from build123d import *

# Parameters (mm, degrees)
CYLINDER1317_R     = 1
CYLINDER1317_DEPTH = 7
CYLINDER1318_R     = 1
CYLINDER1318_DEPTH = 7
CYLINDER1319_R     = 1
CYLINDER1319_DEPTH = 7
CYLINDER1320_R     = 1
CYLINDER1320_DEPTH = 7
BOX543_W           = 4
BOX543_H           = 11
BOX543_DEPTH       = 4
CYLINDER1293_R     = 2
CYLINDER1293_DEPTH = 11
CYLINDER1292_R     = 3
CYLINDER1292_DEPTH = 6.5
CYLINDER1286_R     = 6
CYLINDER1286_DEPTH = 6.5
CYLINDER1310_R     = 13.75
CYLINDER1310_DEPTH = 5
CYLINDER1291_R     = 5.6
CYLINDER1291_DEPTH = 4.5
CYLINDER1290_R     = 10
CYLINDER1290_DEPTH = 6
BOX507_W           = 22
BOX507_H           = 26
BOX507_DEPTH       = 5


with BuildPart() as cylinder1317:
    # Cylinder1317 → Cylinder1317 (new body)
    with BuildSketch(Plane(origin=(439, 96, 121), x_dir=(0, 0, -1), z_dir=(1, 0, 0))):
        Circle(CYLINDER1317_R)
    extrude(amount=CYLINDER1317_DEPTH)


with BuildPart() as fusion248002050190:
    # Cylinder1318 → Cylinder1318 (new body)
    with BuildSketch(Plane(origin=(439, 74, 121), x_dir=(0, 0, -1), z_dir=(1, 0, 0))):
        Circle(CYLINDER1318_R)
    extrude(amount=CYLINDER1318_DEPTH)

    # Fusion248002050190: union Cylinder1317
    add(cylinder1317.part)


with BuildPart() as fusion248002050190_1:
    # Fusion248002050190 placement: moved
    add(fusion248002050190.part.moved(Location((12, 0, 7))))


with BuildPart() as cylinder1319:
    # Cylinder1319 → Cylinder1319 (new body)
    with BuildSketch(Plane(origin=(439, 96, 121), x_dir=(0, 0, -1), z_dir=(1, 0, 0))):
        Circle(CYLINDER1319_R)
    extrude(amount=CYLINDER1319_DEPTH)


with BuildPart() as fusion248002050192:
    # Cylinder1320 → Cylinder1320 (new body)
    with BuildSketch(Plane(origin=(439, 74, 121), x_dir=(0, 0, -1), z_dir=(1, 0, 0))):
        Circle(CYLINDER1320_R)
    extrude(amount=CYLINDER1320_DEPTH)

    # Fusion248002050191: union Cylinder1319
    add(cylinder1319.part)


with BuildPart() as fusion248002050192_1:
    # Fusion248002050191 placement: moved
    add(fusion248002050192.part.moved(Location((27, 0, 7))))

    # Fusion248002050192: union Fusion248002050190
    add(fusion248002050190_1.part)


with BuildPart() as cube769:
    # Box543 → Box543 (new body)
    with BuildSketch(Plane(origin=(460, 88, 128), x_dir=(1, 0, 0), z_dir=(0, 0, 1))):
        with Locations((2, 5.5)):
            Rectangle(BOX543_W, BOX543_H)
    extrude(amount=BOX543_DEPTH)


with BuildPart() as fusion248002050172:
    # Cylinder1293 → Cylinder1293 (new body)
    with BuildSketch(Plane(origin=(462, 88, 128), x_dir=(1, 0, 0), z_dir=(0, 1, 0))):
        Circle(CYLINDER1293_R)
    extrude(amount=CYLINDER1293_DEPTH)

    # Fusion248002050172: union Cube769
    add(cube769.part)


with BuildPart() as cylinder1292:
    # Cylinder1292 → Cylinder1292 (new body)
    with BuildSketch(Plane(origin=(462, 85, 123), x_dir=(1, 0, 0), z_dir=(0, 0, 1))):
        Circle(CYLINDER1292_R)
    extrude(amount=CYLINDER1292_DEPTH)


with BuildPart() as cylinder1286:
    # Cylinder1286 → Cylinder1286 (new body)
    with BuildSketch(Plane(origin=(462, 85, 125), x_dir=(1, 0, 0), z_dir=(0, 0, 1))):
        Circle(CYLINDER1286_R)
    extrude(amount=CYLINDER1286_DEPTH)


with BuildPart() as cylinder1310:
    # Cylinder1310 → Cylinder1310 (new body)
    with BuildSketch(Plane(origin=(462, 85, 125), x_dir=(1, 0, 0), z_dir=(0, 0, 1))):
        Circle(CYLINDER1310_R)
    extrude(amount=CYLINDER1310_DEPTH)


with BuildPart() as cylinder1291:
    # Cylinder1291 → Cylinder1291 (new body)
    with BuildSketch(Plane(origin=(462, 85, 119.5), x_dir=(1, 0, 0), z_dir=(0, 0, 1))):
        Circle(CYLINDER1291_R)
    extrude(amount=CYLINDER1291_DEPTH)


with BuildPart() as cut014301:
    # Cylinder1290 → Cylinder1290 (new body)
    with BuildSketch(Plane(origin=(462, 85, 119.5), x_dir=(1, 0, 0), z_dir=(0, 0, 1))):
        Circle(CYLINDER1290_R)
    extrude(amount=CYLINDER1290_DEPTH)

    # Cut014301: cut Cylinder1291
    add(cylinder1291.part, mode=Mode.SUBTRACT)


with BuildPart() as bucket_head:
    # Box507 → Box507 (new body)
    with BuildSketch(Plane(origin=(451, 72, 125), x_dir=(1, 0, 0), z_dir=(0, 0, 1))):
        with Locations((11, 13)):
            Rectangle(BOX507_W, BOX507_H)
    extrude(amount=BOX507_DEPTH)

    # Fusion248002050171: union Cut014301
    add(cut014301.part)

    # Fusion248002050186: union Cylinder1310
    add(cylinder1310.part)

    # Cut014314: cut Cylinder1286
    add(cylinder1286.part, mode=Mode.SUBTRACT)

    # Cut014315: cut Cylinder1292
    add(cylinder1292.part, mode=Mode.SUBTRACT)

    # Cut014316: cut Fusion248002050172
    add(fusion248002050172.part, mode=Mode.SUBTRACT)

    # Cut014318: cut Fusion248002050192
    add(fusion248002050192_1.part, mode=Mode.SUBTRACT)


solid = bucket_head.part
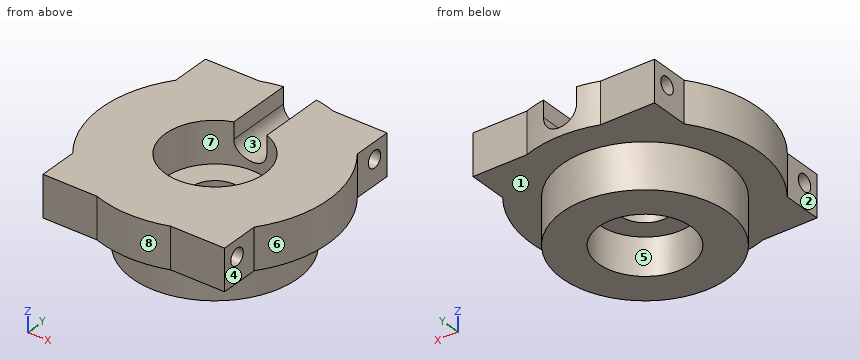
The model under review builds one solid part; all positions refer to its coordinate system, in mm. Face numbers are marked on the shaded views. A direction names the side the tool comes from. Coordinates: 2 decimals unless noted, no trailing zeros. Loops run counter-clockwise (first coordinate to the right, second up) from the corner with the lowest first, then second, coordinate; pieces in that order, holes last. Notation, with made-up numbers: M 45.5,-11.5 L 84.5,-11.5 A27 ccw 84.5,9.5 Z; hole C 77,-37.75 d5. An arc over 180 degrees is marked long. Put each result on its own line as item: value. Start each with the question number.
Q1. Add section A-A (x = 462). Write out the cut boundary in (y, z), and give its area (3 significant figures).
Q2. Add section B-B (y = 74). Write out the cut boundary in (x, z).
Q3. Add section C-C (z = 123). Write out the cut boundary in (x, y), and give its area (3 significant figures).
Q4. Clearance check with flat-ended pins moving along their axes: pin 1 (6 mm diameter, centred on x = 462, z = 120.5, fed in from -Y); pin 2 (0.6 mm diameter, centred on y = 74, z = 128, fed in from -X); pin 3 (2 mm diameter, centred on y = 95.5, z = 129, fed in from +X). State where each tip first meets the part, or that it passes through.
Q5. Wall thickness on line 1 (Y direction, x = 454.25, z = 128); line 2 (Z direction, x = 454.5, y = 96); line 3 (X direction, y = 85, z = 128.35): over which ranges is each line inside the solid? List them lowest first.
Q6. For the marked faces 1, 2, 3 and 4, list the 3-axis set-ups (+Z, -Z, +X, -X, +Y, -Y) from which the entire face can be reached by the end or side of a thin tool; tool diameter is ignored.
Q7. The part is to be moulded in two halves that separate along X. For the marked faces 5, 6, 7 and 8, say which applies: +X half, -X half, draft (parallel to the pull), parting line (faces both ways), or undercut.
Q8. Add section D-D (x = 469.25). Write out the cut boundary in (y, z), and give its area (3 significant figures).
Answers:
1. outline: M 71.25,125 L 75,125 L 75,119.5 L 79.4,119.5 L 79.4,124 L 82,124 L 82,125 L 79,125 L 79,130 L 71.25,130 Z; M 88,124 L 90.6,124 L 90.6,119.5 L 95,119.5 L 95,125 L 98.75,125 L 98.75,126 L 91,126 L 91,125 L 88,125 Z
1. area: 100 mm^2
2. outline: M 451,125 L 473,125 L 473,127 L 466,127 L 466,129 L 473,129 L 473,130 L 451,130 L 451,129 L 458,129 L 458,127 L 451,127 Z
3. outline: C 462,85 d20; hole C 462,85 d11.2
3. area: 216 mm^2
4. pin 1: stops at y = 75
4. pin 2: stops at x = 458
4. pin 3: stops at x = 473
5. line 1: y = 72 to 73, 75 to 95, 97 to 98
5. line 2: z = 125 to 127, 129 to 130
5. line 3: x = 448.25 to 456, 468 to 475.75
6. face 1: -Z
6. face 2: +Z, -Z, -X, -Y
6. face 3: +Z, +Y
6. face 4: +Z, -Z, +X, -Y
7. face 5: undercut
7. face 6: +X half
7. face 7: undercut
7. face 8: parting line
8. outline: M 72,125 L 78.11,125 L 78.11,119.5 L 91.89,119.5 L 91.89,125 L 98,125 L 98,130 L 72,130 Z; hole C 74,128 d2; hole C 96,128 d2
8. area: 199 mm^2
